Autodesk Inventor part; units mm, degrees
ref_plane "YZ Plane" through (0, 0, 0) normal (1, 0, 0) x (0, 1, 0)
ref_plane "XZ Plane" through (0, 0, 0) normal (0, 1, 0) x (-1, 0, 0)
ref_plane "XY Plane" through (0, 0, 0) normal (0, 0, 1) x (1, 0, 0)
sketch "Sketch1" plane through (0, 0, 0) normal (0, 0, 1) x (1, 0, 0)
  line L0 (-10, -10) -> (10, -10)
  line L1 (10, -10) -> (10, 10)
  line L2 (10, 10) -> (-10, 10)
  line L3 (-10, 10) -> (-10, -10)
  line L4 (-10, -10) -> (10, 10) construction
  line L5 (10, -10) -> (-10, 10) construction
  point P0 (0, 0)
  dimension "d0" = 20
  dimension "d1" = 20
extrude "Extrusion1" add sketch "Sketch1" along normal blind 20
sketch "Sketch2" plane through (-10, 10, 0) normal (0, 1, 0) x (1, 0, 0)
  circle A0 centre (10, -10) radius 7.6
  line L0 (0, 0) -> (0, -20)
  point P0 (10, 0)
  dimension "d4" = 15.2
  dimension "d5" = 10
  dimension "d6" = 10
extrude "Extrusion2" cut sketch "Sketch2" against normal blind 2
sketch "Sketch3" plane through (0, 0, 0) normal (0, 0, -1) x (-1, 0, 0)
  circle A0 centre (0, 0) radius 7.6
  dimension "d9" = 15.2
extrude "Extrusion3" cut sketch "Sketch3" against normal blind 2
sketch "Sketch4" plane through (-10, -10, 0) normal (-1, 0, 0) x (0, 0, 1)
  circle A0 centre (10, 10) radius 7.6
  line L0 (0, 20) -> (0, 0)
  line L1 (0, 20) -> (20, 20)
  point P0 (0, 10)
  dimension "d12" = 15.2
  dimension "d13" = 10
  dimension "d14" = 10
extrude "Extrusion4" cut sketch "Sketch4" against normal blind 2
fillet "Fillet1" radius 2 11 edges at (-10, 10, 10) (0, 10, 20) (-10, 0, 20) (-10, 0, 0) (0, -10, 0) (10, 0, 0) (0, 10, 0) (10, 10, 10) (10, -10, 10) (0, -10, 20) (10, 0, 20)
sketch "Sketch5" plane through (-8, 0, 10) normal (-1, 0, 0) x (0, 0, 1)
  circle A0 centre (0, 0) radius 4.07
  point P0 (-10, 0)
  dimension "d18" = 8.14
extrude "Extrusion5" cut sketch "Sketch5" against normal blind 3.5
sketch "Sketch6" plane through (0, 0, 2) normal (0, 0, -1) x (-1, 0, 0)
  circle A0 centre (0, 0) radius 3.98
  dimension "d21" = 7.96
extrude "Extrusion6" cut sketch "Sketch6" against normal blind 3.5
sketch "Sketch7" plane through (0, 8, 10) normal (0, 1, 0) x (1, 0, 0)
  circle A0 centre (0, 0) radius 4.07
  point P0 (0, 10)
  dimension "d24" = 8.14
extrude "Extrusion7" cut sketch "Sketch7" against normal blind 3.5
fillet "Fillet2" radius 2 3 edges at (-9.4142, -9.4142, 19.4142) (-9.4142, -9.4142, 0.5858) (-10, -10, 10)
fillet "Fillet3" radius 1 1 edges at (-8, 0, 5.93)
fillet "Fillet4" radius 1 1 edges at (-4.07, 8, 10)
fillet "Fillet5" radius 1 1 edges at (3.98, 0, 2)
equation "\"d1\" = d0"
equation "\"d6\" = d5"
equation "\"d13\" = d14"
properties part number "Center"
Verification items for the finished model (mm, model axes). A direction names the side the tool comes from. Coordinates: 2 decimals unless noted, no trailing zeros. Order: outer loops, then holes, each group sorted by start corner. A loop starts at its lowest first (then second) coordinate and runs counter-clockwise, first axis right, second up.
Item 1: Access from +Z, -Z, +X, -X, +Y, -Y to the whole of each face (thin tool, end or side, straight path). Record for faces 5 (the face through (-9.4, -9.43, 9.89)), 6 (the face through (-9.01, -2.91, 17.02)), 7 (the face through (0, 4.5, 10)).
Filled in:
face 5: +Z, -Z, -X, -Y
face 6: -X
face 7: +Y
Item 2: Section check C-C, the plane x = 6.5. Enter the section's corners in (y, z), then the cut area to 3 significant figures.
Filled in:
outline: (-10, 2) arc R2 ccw to (-8, 0) - (-3.94, 0) - (-3.94, 2) - (3.94, 2) - (3.94, 0) - (8, 0) arc R2 ccw to (10, 2) - (10, 6.06) - (8, 6.06) - (8, 13.94) - (10, 13.94) - (10, 18) arc R2 ccw to (8, 20) - (-8, 20) arc R2 ccw to (-10, 18) - close
area: 365 mm2
Item 3: Depth check by flat-ended pin: pin 1 (5 mm diameter, centred on y = 0, z = 10, fed in from -X); pin 2 (4.5 mm diameter, centred on y = -0.5, z = 7, fed in from -X); pin 3 (4.5 mm diameter, centred on x = 0.5, y = 1.5, fed in from -Z). Enter the tip coordinate at first touch or a pass-through.
Filled in:
pin 1: stops at x = -4.5
pin 2: stops at x = -8
pin 3: stops at z = 5.5
Item 4: Section check A-A, the plane y = 0. Enter the section's corners in (x, z), then the cut area to 3 significant figures.
Filled in:
outline: (-10, 2) arc R2 ccw to (-8, 0) - (-7.6, 0) - (-7.6, 2) - (-4.98, 2) arc R1 ccw to (-3.98, 3) - (-3.98, 5.5) - (3.98, 5.5) - (3.98, 3) arc R1 ccw to (4.98, 2) - (7.6, 2) - (7.6, 0) - (8, 0) arc R2 ccw to (10, 2) - (10, 18) arc R2 ccw to (8, 20) - (-8, 20) arc R2 ccw to (-10, 18) - (-10, 17.6) - (-8, 17.6) - (-8, 15.07) arc R1 ccw to (-7, 14.07) - (-4.5, 14.07) - (-4.5, 5.93) - (-7, 5.93) arc R1 ccw to (-8, 4.93) - (-8, 2.4) - (-10, 2.4) - close
area: 279 mm2
Item 5: Material ranges on L1, parallel to Z at x = 0, y = 5.5; L2, parallel to X at y = 2.75, z = 11.5; L3, parallel to X at y = -5, z = 8.5, recorded low to high.
Filled in:
L1: z = 2 to 5.93, 14.07 to 20
L2: x = -4.5 to 10
L3: x = -8 to 10
Item 6: Release check for a two-part mould opening along Y. For faces 1 (the face through (0, -10, 10)), 2 (the face through (-9.43, -0.11, 0.6)), 3 (the face through (-4.5, 0, 10)), 4 (the face through (7.593, 0.334, 0.986)) record: +Y half, -Y half, draft (parallel to the pull), parting line (faces both ways), or undercut.
Filled in:
face 1: -Y half
face 2: draft
face 3: undercut
face 4: undercut
Item 7: Section check B-B, the plane z = 10. Enter the section's corners in (x, y).
Filled in:
outline: (-10, -8) arc R2 ccw to (-8, -10) - (8, -10) arc R2 ccw to (10, -8) - (10, 8) arc R2 ccw to (8, 10) - (7.6, 10) - (7.6, 8) - (5.07, 8) arc R1 ccw to (4.07, 7) - (4.07, 4.5) - (-4.07, 4.5) - (-4.07, 7) arc R1 ccw to (-5.07, 8) - (-7.6, 8) - (-7.6, 10) - (-8, 10) arc R2 ccw to (-10, 8) - (-10, 7.6) - (-8, 7.6) - (-8, 5.07) arc R1 ccw to (-7, 4.07) - (-4.5, 4.07) - (-4.5, -4.07) - (-7, -4.07) arc R1 ccw to (-8, -5.07) - (-8, -7.6) - (-10, -7.6) - close
Item 8: Section check D-D, the plane x = -6.5. Enter the section's corners in (y, z), then the cut area to 3 significant figures.
Filled in:
outline: (-10, 2) arc R2 ccw to (-8, 0) - (-3.94, 0) - (-3.94, 2) - (3.94, 2) - (3.94, 0) - (8, 0) arc R2 ccw to (10, 2) - (10, 6.06) - (8, 6.06) - (8, 13.94) - (10, 13.94) - (10, 18) arc R2 ccw to (8, 20) - (-8, 20) arc R2 ccw to (-10, 18) - close; hole circle Ø8.14 at (0, 10)
area: 313 mm2
